Check sheet for the modelled part. Datum: model origin and axes. Units: mm. A direction names the side the tool comes from. Round coordinates to 2 decimals unless told otherwise and drop trailing zeros. Write each loop counter-clockwise with the first axis right and the second up, starting at its lowest first coordinate (ties: lowest second). Pieces come first, ordered by that corner, then holes. Notation, with made-up numbers: (-20.75, 47) -> (5.25, 47) arc R32 ccw to (5.25, 79) -> close; hole circle Ø1 at (34.25, 78). An arc over 180 degrees is marked (long way). One line per item, written item: value.
Autodesk Inventor part; units mm, degrees
ref_plane "YZ Plane" through (0, 0, 0) normal (1, 0, 0) x (0, 1, 0)
ref_plane "XZ Plane" through (0, 0, 0) normal (0, 1, 0) x (-1, 0, 0)
ref_plane "XY Plane" through (0, 0, 0) normal (0, 0, 1) x (1, 0, 0)
sketch "Sketch1" plane through (0, 0, 0) normal (0, 1, 0) x (-1, 0, 0)
  circle A0 centre (0, 0) radius 30.5
  circle A1 centre (0, 0) radius 28.75
  line L0 (18.166, -27.5) -> (-18.166, -27.5)
  line L1 (-18.166, -27.5) -> (-18.166, 27.5)
  line L2 (-18.166, 27.5) -> (18.166, 27.5)
  line L3 (18.166, 27.5) -> (18.166, -27.5)
  line L4 (18.166, -27.5) -> (-18.166, 27.5) construction
  line L5 (-18.166, -27.5) -> (18.166, 27.5) construction
  line L6 (26.5, -26.5) -> (-26.5, -26.5)
  line L7 (-26.5, -26.5) -> (-26.5, 26.5)
  line L8 (-26.5, 26.5) -> (26.5, 26.5)
  line L9 (26.5, 26.5) -> (26.5, -26.5)
  line L10 (26.5, -26.5) -> (-26.5, 26.5) construction
  line L11 (-26.5, -26.5) -> (26.5, 26.5) construction
  point P0 (11.1496, -26.5)
  point P1 (-11.1496, -26.5)
  point P2 (-11.1496, 26.5)
  point P3 (11.1496, 26.5)
  point P4 (18.166, -24.4999)
  point P5 (18.166, 24.4999)
  point P6 (-18.166, 24.4999)
  point P7 (-18.166, -24.4999)
  dimension "d0" = 61
  dimension "d1" = 1.75
  dimension "d4" = 36.332
  dimension "d5" = 55
  dimension "d6" = 53
  dimension "d7" = 53
extrude "Extrusion1" add sketch "Sketch1" along normal blind 2 contours A0 L9 A1 | L9 A1 L3 A0 | A0 L3 A1 L9 | L3 A1 L8 A0 | A0 L8 L3 | L3 L6 A0 | A0 L6 A1 L3 | L8 A1 L2 A0 | A0 L2 L3 L8 | L6 L3 L0 A0 | A0 L0 A1 L6 | L8 A1 L2 | A1 L0 L6 | L2 A1 L8 A0 | A0 L8 L1 L2 | A1 L1 A0 L8 | L0 L1 L6 A0 | A0 L6 A1 L0 | L6 A0 L1 A1 | A0 L1 L8 | A1 L7 A0 L1 | L6 L1 A0 | L1 A0 L7 A1 | A1 L7 A0
sketch "Sketch2" plane through (0, 2, 0) normal (0, 1, 0) x (1, 0, 0)
  line L0 (-18.166, -27.5) -> (18.166, -27.5)
  line L1 (11.1496, -26.5) -> (-11.1496, -26.5)
  line L2 (1.8, -27.5) -> (-1.8, -27.5)
  line L3 (-1.8, -27.5) -> (-1.8, -26.5)
  line L4 (-1.8, -26.5) -> (1.8, -26.5)
  line L5 (1.8, -26.5) -> (1.8, -27.5)
  point P0 (0, 0)
  point P1 (0, -26.5)
  point P2 (1.8, -27)
  dimension "d8" = 3.6
  dimension "d9" = 1.8
extrude "Extrusion2" add sketch "Sketch2" along normal blind 9
mirror "Mirror1" about plane through (0, 0, 0) normal (0, 0, 1) of "Extrusion2"
properties part number "cir"
Item 1: Depth check by flat-ended pin: pin 1 (2 mm diameter, centred on y = 1, z = -26, fed in from -X); pin 2 (2 mm diameter, centred on y = 1, z = -26.5, fed in from +X); pin 3 (0.8 mm diameter, centred on y = 7, z = -27, fed in from -X); pin 4 (1 mm diameter, centred on y = 3.5, z = 20, fed in from -X). Enter the tip coordinate at first touch or a pass-through.
Result set:
pin 1: x = -18.17
pin 2: x = 18.17
pin 3: x = -1.8
pin 4: through
Item 2: Release check for a two-part mould opening along X. For faces 6 (the cylindrical face through (30.497, 0.986, -0.398)), 7 (the flat face through (0, 3, 27.5)), 8 (the flat face through (0, 4, -26.5)), 9 (the cylindrical face through (28.746, 0.986, -0.472)) record: pulls with the +X half, pulls with the -X half, needs draft (parallel to the pull), parting line crosses it, or undercut.
Result set:
face 6: pulls with the +X half
face 7: needs draft
face 8: undercut
face 9: undercut
Item 3: Sectioned sample at B-B (x = -9). Enter the section's corners in (y, z), then the cut area to 3 significant figures.
Result set:
outline: (0, -27.5) -> (2, -27.5) -> (2, -26.5) -> (0, -26.5) -> close; (0, 26.5) -> (2, 26.5) -> (2, 27.5) -> (0, 27.5) -> close
area: 4.00 mm^2
Item 4: Tool access check on faces 1 (the flat face through (0, 4, 26.5)), 2 (the flat face through (-18.166, 1, 26)), 3 (the flat face through (18.166, 1, -26)), 4 (the flat face through (29, 2, 2)), 5 (the flat face through (-29, 2, 4)). Record the directions out of +Z, -Z, +X, -X, +Y, -Y that give a thin tool (end or side, any length) a straight path to the whole face; none if there is none.
Result set:
face 1: +Y, -Y
face 2: +Z, -X, +Y, -Y
face 3: -Z, +X, +Y, -Y
face 4: +Z, -Z, +X, +Y
face 5: +Z, -Z, -X, +Y
Item 5: Material ranges on line 1 along X through (y, z) = (1.5, 0.5); line 2 along X through (y, z) = (1, 17), recorded low to high.
Result set:
line 1: -30.5 to -28.75, 28.75 to 30.5
line 2: -25.32 to -23.19, 23.19 to 25.32
Item 6: Sectioned sample at A-A (y = 5). Enter the section's corners in (x, z).
Result set:
outline: (-1.8, -27.5) -> (1.8, -27.5) -> (1.8, -26.5) -> (-1.8, -26.5) -> close; (-1.8, 26.5) -> (1.8, 26.5) -> (1.8, 27.5) -> (-1.8, 27.5) -> close
